Autodesk Inventor part; units mm, degrees
ref_plane "YZ Plane" through (0, 0, 0) normal (1, 0, 0) x (0, 1, 0)
ref_plane "XZ Plane" through (0, 0, 0) normal (0, 1, 0) x (-1, 0, 0)
ref_plane "XY Plane" through (0, 0, 0) normal (0, 0, 1) x (1, 0, 0)
sketch "Sketch1" plane through (0, 0, 0) normal (0, 1, 0) x (-1, 0, 0)
  line L0 (8, 7.5) -> (-8, 7.5)
  line L1 (-8, 7.5) -> (-8, -7.5)
  line L2 (-8, -7.5) -> (8, -7.5)
  line L3 (8, -7.5) -> (8, 7.5)
  point P0 (0, 0)
  dimension "d0" = 15
  dimension "d1" = 7.5
  dimension "d2" = 16
  dimension "d3" = 8
extrude "Extrusion1" add sketch "Sketch1" along normal blind 8.5
fillet "Fillet1" radius 1 2 edges at (-8, 4.25, 7.5) (-8, 4.25, -7.5)
sketch "Sketch2" plane through (8, 0, 7.5) normal (0, 0, 1) x (1, 0, 0)
  line L0 (0, 0) -> (0, 8.5)
  line L1 (0, 1) -> (3, 1)
  line L2 (3, 1) -> (3, 1.8)
  line L3 (3, 1.8) -> (0, 1.8)
  line L4 (0, 1.8) -> (0, 1)
  line L5 (-15, 8.5) -> (0, 8.5)
  line L6 (-16, 8.5) -> (-16, 0)
  point P0 (-8, 0)
  dimension "d7" = 0.8
  dimension "d8" = 6.7
  dimension "d9" = 19
extrude "Extrusion2" add sketch "Sketch2" against normal blind 15
sketch "Sketch3" plane through (8, 1.8, 7.5) normal (0, 1, 0) x (1, 0, 0)
  circle A0 centre (1.6, 6.865) radius 0.25
  line L0 (0, 0) -> (0, 15) construction
  line L1 (0, 9.8681) -> (0, 6.3547)
  circle A1 centre (1.6, 8.135) radius 0.25
  circle A2 centre (1.6, 9.405) radius 0.25
  circle A3 centre (1.6, 10.675) radius 0.25
  circle A4 centre (1.6, 5.595) radius 0.25
  circle A5 centre (1.6, 4.325) radius 0.25
  point P0 (-8, 7.5)
  dimension "d12" = 0.5
  dimension "d13" = 9.6
  dimension "d15" = 0.635
  dimension "d18" = 1.27
  dimension "d25" = 1.27
extrude "Extrusion3" cut sketch "Sketch3" against normal blind 15
sketch "Sketch4" plane through (0, 8.5, 0) normal (0, 1, 0) x (1, 0, 0)
  line L0 (-2.1812, 4.05) -> (2.1812, 4.05)
  line L1 (2.1812, -4.05) -> (-2.1812, -4.05)
  arc A0 (-2.1812, 4.05) -> (-2.1812, -4.05) centre (0, 0) ccw
  arc A1 (2.1812, -4.05) -> (2.1812, 4.05) centre (0, 0) ccw
  dimension "d33" = 4.05
  dimension "d34" = 8.1
extrude "Extrusion4" add sketch "Sketch4" along normal blind 8
sketch "Sketch5" plane through (0, 16.5, 0) normal (0, 1, 0) x (1, 0, 0)
  circle A0 centre (0, 0) radius 3.2
  dimension "d37" = 6.4
extrude "Extrusion5" add sketch "Sketch5" along normal blind 2.5
sketch "Sketch6" plane through (0, 19, 0) normal (0, 1, 0) x (1, 0, 0)
  circle A0 centre (0, 0) radius 3.15
  dimension "d40" = 6.3
extrude "Extrusion6" add sketch "Sketch6" along normal blind 0.65
sketch "Sketch7" plane through (0, 19.65, 0) normal (0, 1, 0) x (1, 0, 0)
  arc A0 (2.41, 2.0284) -> (2.41, -2.0284) centre (0, 0) ccw
  line L0 (2.41, -2.0284) -> (2.41, 2.0284)
  dimension "d43" = 6.3
  dimension "d44" = 5.56
extrude "Extrusion7" add sketch "Sketch7" along normal blind 6.35
properties part number "C14D32P-A3_Encoder"
Source: CAD feature listing. Evaluate the final solid. Frame: model axes, mm. A direction names the side the tool comes from. Coordinates: 2 decimals unless noted, no trailing zeros. Loops run counter-clockwise (first coordinate to the right, second up) from the corner with the lowest first, then second, coordinate; pieces in that order, holes last. Notation, with made-up numbers: (34, 63) -> (49, 63) arc R17 ccw to (49, 70) -> close; hole circle Ø1 at (-26.5, 6.25). An arc over 180 degrees is marked (long way). Answer in a Markdown table with one row per item. Add a question column.
Q1. Section A-A on z = -4.5. Return the cut outline in (x, y), and give its area (3 significant figures).
Q2. Ray query, line 1 along Y through (x, z) = (-3.5, 1.25); line 2 along Y through (x, z) = (6.25, -6.5); line 3 along X through (y, z) = (6.75, 3). Return the intervals inside material, ascending.
Q3. Section C-C on y = 18.5. Return the cut outline in (x, z), and give its area (3 significant figures).
Q4. Section B-B on x = 0. Return the cut outline in (y, z), and give its area (3 significant figures).
Q5. Section D-D on z = 0. Return the cut outline in (x, y), and give its area (3 significant figures).
Q6. Contact query for flat-ended pins moving along their axis: pin 1 Ø4.5 at (y, z) = (22, 0.5) entering from +X; pin 2 Ø7.5 at (x, z) = (3.5, 1.5) entering from +Y; pin 3 Ø2 at (x, z) = (-1, 4.5) entering from +Y; pin 4 Ø2.5 at (x, z) = (9.5, -3.5) entering from +Y. Output: stop coordinate, or through.
Q7. Reachability of faces 1 (the face through (0, 12, -4.05)), 2 (the face through (10, 1.8, 0)), 3 (the face through (-2.539, 17.732, -1.947)) from +Z, -Z, +X, -X, +Y, -Y: full face, straight path, thin tool, end or side. Return the list, or none.
Computed values:
| question | item | result |
|---|---|---|
| 1 | outline | (-8, 0) -> (8, 0) -> (8, 1) -> (11, 1) -> (11, 1.8) -> (8, 1.8) -> (8, 8.5) -> (-8, 8.5) -> close |
| 1 | area | 138 mm^2 |
| 2 | line 1 | y = 0 to 16.5 |
| 2 | line 2 | y = 0 to 8.5 |
| 2 | line 3 | x = -8 to 8 |
| 3 | outline | circle Ø6.4 at (0, 0) |
| 3 | area | 32.2 mm^2 |
| 4 | outline | (0, -7.5) -> (8.5, -7.5) -> (8.5, -4.05) -> (16.5, -4.05) -> (16.5, -3.2) -> (19, -3.2) -> (19, -3.15) -> (26, -3.15) -> (26, 3.15) -> (19, 3.15) -> (19, 3.2) -> (16.5, 3.2) -> (16.5, 4.05) -> (8.5, 4.05) -> (8.5, 7.5) -> (0, 7.5) -> close |
| 4 | area | 252 mm^2 |
| 5 | outline | (-8, 0) -> (8, 0) -> (8, 1) -> (11, 1) -> (11, 1.8) -> (8, 1.8) -> (8, 8.5) -> (4.6, 8.5) -> (4.6, 16.5) -> (3.2, 16.5) -> (3.2, 19) -> (3.15, 19) -> (3.15, 19.65) -> (2.41, 19.65) -> (2.41, 26) -> (-3.15, 26) -> (-3.15, 19) -> (-3.2, 19) -> (-3.2, 16.5) -> (-4.6, 16.5) -> (-4.6, 8.5) -> (-8, 8.5) -> close |
| 5 | area | 267 mm^2 |
| 6 | pin 1 | stops at x = 2.41 |
| 6 | pin 2 | stops at y = 26 |
| 6 | pin 3 | stops at y = 16.5 |
| 6 | pin 4 | stops at y = 1.8 |
| 7 | face 1 | -Z, +X, -X, +Y |
| 7 | face 2 | +Z, -Z, +X, +Y |
| 7 | face 3 | +Y |
